```python
from build123d import *

# Parameters (mm, degrees)
F1_DEPTH  = 3.175
F2_W      = 1.27
F2_H      = 3.175
F3_DEPTH  = 2.54
F4_W      = 1.27
F4_H      = 3.175
F5_DEPTH  = 2.54
F6_W      = 6.985
F6_H      = 3.175
F7_DEPTH  = 6.35
F9_DEPTH  = 25.4
F10_DEPTH = 25.4


# Not quite as in the source:
# - a feature names something its author has since deleted; it is built from what else it names


with BuildPart() as f1:
    # F0 (on Top) → F1 (new body)
    with BuildSketch(Plane.XY):
        Polygon((0, 63.5), (0, 0), (15.875, 0), (15.875, 12.7), (12.065, 12.7), (12.065, 50.8), (15.875, 50.8), (15.875, 63.5), align=None)
        Polygon((15.875, 12.7), (15.875, 0), (31.75, 0), (31.75, 63.5), (15.875, 63.5), (15.875, 50.8), (19.685, 50.8), (19.685, 12.7), align=None)
    extrude(amount=F1_DEPTH)

    # F2 (on face) → F3 (cut)
    with BuildSketch(Plane.YZ.offset(31.75)):
        with Locations((31.75, 1.5875)):
            Rectangle(F2_W, F2_H)
    extrude(amount=-F3_DEPTH, mode=Mode.SUBTRACT)

    # F4 (on face) → F5 (cut)
    with BuildSketch(Plane(origin=(0, 0, 0), x_dir=(0, -1, 0), z_dir=(-1, 0, 0))):
        with Locations((-31.75, 1.5875)):
            Rectangle(F4_W, F4_H)
    extrude(amount=-F5_DEPTH, mode=Mode.SUBTRACT)

    # F6 (on face) → F7 (join)
    with BuildSketch(Plane.XZ):
        with Locations((3.4925, 1.5875)):
            Rectangle(F6_W, F6_H)
        with Locations((28.2575, 1.5875)):
            Rectangle(F6_W, F6_H)
    extrude(amount=F7_DEPTH)

    # F8 (on face) → F9 (cut)
    with BuildSketch(Plane.XY.offset(3.175)):
        with BuildLine():
            ThreePointArc((5.29375, -4.35), (3.0318335149, -3.4130835149), (3.96875, -5.675))
            Line((3.96875, -5.675), (3.96875, -4.35))
            Line((3.96875, -4.35), (5.29375, -4.35))
        make_face()
        with BuildLine():
            Line((3.96875, -4.35), (3.96875, -5.675))
            ThreePointArc((3.96875, -5.675), (4.9056664851, -5.2869164851), (5.29375, -4.35))
            Line((5.29375, -4.35), (3.96875, -4.35))
        make_face()
        with BuildLine():
            ThreePointArc((27.78125, -3.025), (26.8443335149, -3.4130835149), (26.45625, -4.35))
            Line((26.45625, -4.35), (27.78125, -4.35))
            Line((27.78125, -4.35), (27.78125, -3.025))
        make_face()
    extrude(amount=-F9_DEPTH, mode=Mode.SUBTRACT)

    # F8 (on face) → F10 (cut)
    with BuildSketch(Plane.XY.offset(3.175)):
        with BuildLine():
            ThreePointArc((29.10625, 61.5), (27.78125, 62.825), (26.45625, 61.5))
            ThreePointArc((26.45625, 61.5), (27.78125, 60.175), (29.10625, 61.5))
        make_face()
        with BuildLine():
            ThreePointArc((5.29375, 61.5), (4.9056664851, 62.4369164851), (3.96875, 62.825))
            ThreePointArc((3.96875, 62.825), (3.0318335149, 60.5630835149), (5.29375, 61.5))
        make_face()
        with BuildLine():
            Line((27.78125, -4.35), (26.45625, -4.35))
            ThreePointArc((26.45625, -4.35), (26.8443335149, -5.2869164851), (27.78125, -5.675))
            ThreePointArc((27.78125, -5.675), (28.7181664851, -5.2869164851), (29.10625, -4.35))
            ThreePointArc((29.10625, -4.35), (28.7181664851, -3.4130835149), (27.78125, -3.025))
            Line((27.78125, -3.025), (27.78125, -4.35))
        make_face()
    extrude(amount=-F10_DEPTH, mode=Mode.SUBTRACT)


solid = f1.part
```
Build history of the part. All positions in model axes, mm. A direction names the side the tool comes from. Coordinates: 2 decimals unless noted, no trailing zeros. Order: outer loops, then holes, each group sorted by start corner. A loop starts at its lowest first (then second) coordinate and runs counter-clockwise, first axis right, second up.
Item 1: Mould opens along Y. For faces 1 (the flat face through (1, 31.115, 2)), 2 (the flat face through (3, -6.35, 2)), 3 (the flat face through (0, 13, 2)) say: released by +Y, released by -Y, zero draft, split by the parting line, or undercut.
Filled in:
face 1: undercut
face 2: released by -Y
face 3: zero draft
Item 2: Saw through at A-A on y = 39. List the corners of the cut face in (x, z) (3 decimals).
Filled in:
outline: (0, 0) - (12.065, 0) - (12.065, 3.175) - (0, 3.175) - close; (19.685, 0) - (31.75, 0) - (31.75, 3.175) - (19.685, 3.175) - close
Item 3: Saw through at B-B on x = 17. List the corners of the cut face in (y, z) (3 decimals), then the cut area to 3 significant figures.
Filled in:
outline: (0, 0) - (12.7, 0) - (12.7, 3.175) - (0, 3.175) - close; (50.8, 0) - (63.5, 0) - (63.5, 3.175) - (50.8, 3.175) - close
area: 80.6 mm2
Item 4: Saw through at C-C on z = 1.65. List the corners of the cut face in (x, y) (3 decimals), then the cut area to 3 significant figures.
Filled in:
outline: (0, -6.35) - (6.985, -6.35) - (6.985, 0) - (24.765, 0) - (24.765, -6.35) - (31.75, -6.35) - (31.75, 31.115) - (29.21, 31.115) - (29.21, 32.385) - (31.75, 32.385) - (31.75, 63.5) - (0, 63.5) - (0, 32.385) - (2.54, 32.385) - (2.54, 31.115) - (0, 31.115) - close; hole circle Ø2.65 at (3.969, -4.35); hole circle Ø2.65 at (3.969, 61.5); hole (12.065, 12.7) - (19.685, 12.7) - (19.685, 50.8) - (12.065, 50.8) - close; hole circle Ø2.65 at (27.781, -4.35); hole circle Ø2.65 at (27.781, 61.5)
area: 1,790 mm2
Item 5: Tool access for faces 4 (the flat face through (6.985, -3, 2)), 5 (the flat face through (1, 32.385, 2)), 6 (the flat face through (30, 31.115, 2)): list every direction of +Z, -Z, +X, -X, +Y, -Y with a clear straight run to the whole face (end or side of a thin tool).
Filled in:
face 4: +Z, -Z, -Y
face 5: +Z, -Z, -X
face 6: +Z, -Z, +X
Item 6: Drill centre lines: L1, parallel to X at y = 61.5, z = 2.2; L2, parallel to X at y = -4.35, z = 2.45 (3 decimals); L3, parallel to X at y = 36.5, z = 2.8 (3 decimals). Where is each one in solid material? Low to high.
Filled in:
L1: x = 0 to 2.64, 5.29 to 26.46, 29.11 to 31.75
L2: x = 0 to 2.644, 5.294 to 6.985, 24.765 to 26.456, 29.106 to 31.75
L3: x = 0 to 12.065, 19.685 to 31.75
Item 7: Drop flat-ended pins along their axis: pin 1 Ø1.6 at (x, z) = (20, 2) entering from -Y; pin 2 Ø2.5 at (x, y) = (27.78, 61.5) entering from +Z. Give the stop position or say it passes through.
Filled in:
pin 1: stops at y = 0
pin 2: passes through
